Part model, mm, in its own coordinate system. A direction names the side the tool comes from. Round coordinates to 2 decimals unless told otherwise and drop trailing zeros. Order: outer loops, then holes, each group sorted by start corner. A loop starts at its lowest first (then second) coordinate and runs counter-clockwise, first axis right, second up. Notation, with made-up numbers: (56, 84.5) -> (81, 84.5) arc R21 ccw to (81, 105.5) -> close; hole circle Ø6 at (49, -17.5). An arc over 180 degrees is marked (long way). Return JSON: item names as keys, results as strings. Group by question number.
Autodesk Inventor part; units mm, degrees
ref_plane "YZ Plane" through (0, 0, 0) normal (1, 0, 0) x (0, 1, 0)
ref_plane "XZ Plane" through (0, 0, 0) normal (0, 1, 0) x (-1, 0, 0)
ref_plane "XY Plane" through (0, 0, 0) normal (0, 0, 1) x (1, 0, 0)
sketch "Sketch1" plane through (0, 0, 0) normal (0, 0, 1) x (1, 0, 0)
  circle A0 centre (0, 0) radius 9.5
  dimension "d0" = 19
extrude "Extrusion1" add sketch "Sketch1" along normal blind 25
sketch "Sketch2" plane through (0, 0, 25) normal (0, 0, 1) x (1, 0, 0)
  point P0 (0, 0)
  point P1 (0, 0)
hole "Hole1" at (0, 0, 25) direction (0, 0, -1) diameter 10 depth 8 tip angle 118
sketch "Sketch3" plane through (0, 0, 0) normal (0, 0, -1) x (-1, 0, 0)
  point P0 (0, 0)
  point P1 (0, 0)
hole "Hole2" at (0, 0, 0) direction (0, 0, 1) diameter 12 depth 8 tip angle 118
sketch "Sketch4" plane through (0, 0, 0) normal (0, 1, 0) x (-1, 0, 0)
  line L0 (9.5, 25) -> (-9.5, 25)
  circle A0 centre (0, 20) radius 2
  point P0 (0, 0)
  dimension "d17" = 5
  dimension "d18" = 4
extrude "Extrusion2" cut sketch "Sketch4" along normal through all
properties part number "handleAdapter"
(1) Probe L1, parallel to Y at x = 0, z = 5.25; L2, parallel to Z at x = 0, y = 6.5; L3, parallel to Y at x = -1.5, z = 18. List the from-to ranges inside material, lowest first. Write a range as [from, to].
(2) Saw through at C-C, the plane x = 7.5. List the corners of the cut face in (y, z).
(3) Saw through at B-B, the plane y = 8.5. List the corners of the cut face in (x, z).
(4) Tool access for faces 4 (the flat face through (4, -4, 25)), 5 (the cylindrical face through (0, -6, 4)), 6 (the cylindrical face through (1.915, -4.619, 20.944)), 7 (the cylindrical face through (2, 7, 20)): list every direction of +Z, -Z, +X, -X, +Y, -Y with a clear straight run to the whole face (end or side of a thin tool).
(5) Saw through at D-D, the plane z = 21.5. List the corners of the cut face in (x, y).
(6) Saw through at A-A, the plane z = 3. List the corners of the cut face in (x, y).
(7) Mould opens along Y. For faces 1 (the conical face through (-0.85, 0.19, 14.52)), 2 (the flat face through (-0.1, -6.2, 0)), 3 (the cylindrical face through (4.38, 8.43, 12.32)) say: pulls with the +Y half, pulls with the -Y half, needs draft (parallel to the pull), parting line crosses it, or undercut.
(8) Pin check, flat tips, straight feed: P1, Ø9.5, axis at x = 0, y = 0, coming from the +Z side; P2, Ø1.5, axis at y = -6.5, z = 12.5, coming from the +X side; P3, Ø1.5, axis at x = -0.5, y = 2, coming from the +Z side. Stop position of each tip, or through.
Results are:
{
 "1": {"L1": "y = [-9.5, -6], [6, 9.5]", "L2": "z = [0, 18], [22, 25]", "L3": "y = [-9.38, -4.77], [4.77, 9.38]"},
 "2": {"outline": "(-5.83, 0) -> (5.83, 0) -> (5.83, 25) -> (-5.83, 25) -> close"},
 "3": {"outline": "(-4.24, 0) -> (4.24, 0) -> (4.24, 25) -> (-4.24, 25) -> close; hole circle Ø4 at (0, 20)"},
 "4": {"face 4": "+Z, +X, -X, +Y, -Y", "face 5": "-Z", "face 6": "+Z", "face 7": "+Y"},
 "5": {"outline": "(-1.32, 4.82) -> (-1.32, 9.41) arc R9.5 ccw (long way) to (1.32, 9.41) -> (1.32, 4.82) arc R5 cw (long way) to start"},
 "6": {"outline": "circle Ø19 at (0, 0); hole circle Ø12 at (0, 0)"},
 "7": {"face 1": "undercut", "face 2": "needs draft", "face 3": "parting line crosses it"},
 "8": {"P1": "stops at z = 16.85", "P2": "stops at x = 7.56", "P3": "stops at z = 15.69"}
}
